Check sheet for the modelled part. Datum: model origin and axes. Units: mm. Face numbers are marked on the shaded views. A direction names the side the tool comes from. Coordinates: 2 decimals unless noted, no trailing zeros. Write each question's results on one line, items separated by ' | '. Start each with the question number.
1. Thickness scan on line 1 (Z direction, x = -0.5, y = -3.75); line 2 (X direction, y = 5, z = 14); line 3 (X direction, y = -1.5, z = 11). Record the ranges inside material, lowest first. Write a range as [from, to].
2. Gauge pin test, flat ends, axial feed: P1, Ø1, axis at y = -6, z = 10, coming from the +X side; P2, Ø1.5, axis at x = 7, y = 7.5, coming from the -Z side; P3, Ø1.5, axis at y = 6, z = 8.5, coming from the +X side. Record the tip position at first contact, or that the pin passes through.
3. Draft check along X on the marked faces 3, 4 and 5. Enter one of: released by +X, released by -X, zero draft, split by the parting line, or undercut.
4. Tool access check on the marked faces 1 and 2. Record the directions out of +Z, -Z, +X, -X, +Y, -Y that give a thin tool (end or side, any length) a straight path to the whole face; none if there is none.
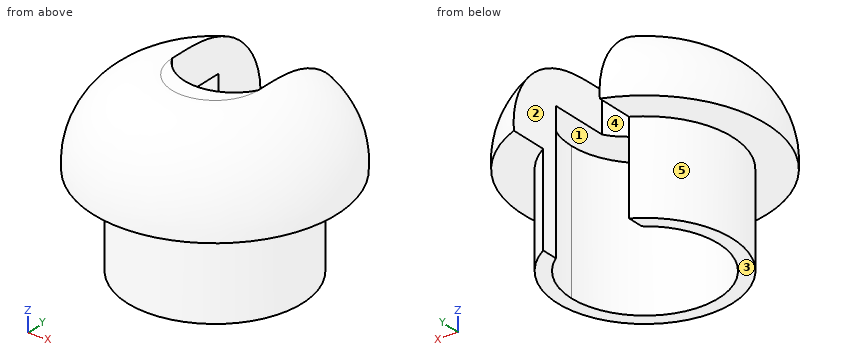
```python
from build123d import *

# Parameters (mm, degrees)
F4_DEPTH = 15.4777297208
F6_DEPTH = 12


with BuildPart() as f2:
    # F1 (on Front) → F2 (revolve)
    with BuildSketch(Plane.XZ):
        with BuildLine():
            Line((0, 15.4767297208), (0, 0))
            Line((0, 0), (7.625, 0))
            Line((7.625, 0), (7.625, 8))
            Line((7.625, 8), (10.625, 8))
            ThreePointArc((10.625, 8), (8.8302197506, 13.2471744611), (3.752507735, 15.4767297208))
            Line((3.752507735, 15.4767297208), (0, 15.4767297208))
        make_face()
    revolve(axis=Axis((0, 0, 0), (0, 0, 1)))

    # F3 (on face) → F4 (cut, through all)
    with BuildSketch(Plane.XY.offset(15.4767297208)):
        with BuildLine():
            ThreePointArc((-3.752507735, 0), (0, -2.1712493207), (3.752507735, 0))
            ThreePointArc((3.752507735, 0), (0, 3.752507735), (-3.752507735, 0))
        make_face()
        with BuildLine():
            Line((3.752507735, 0), (3.752507735, 9.9402872543))
            ThreePointArc((3.752507735, 9.9402872543), (0, 10.625), (-3.752507735, 9.9402872543))
            Line((-3.752507735, 9.9402872543), (-3.752507735, 0))
            ThreePointArc((-3.752507735, 0), (0, 3.752507735), (3.752507735, 0))
        make_face()
        with BuildLine():
            ThreePointArc((-3.752507735, 9.9402872543), (0, 10.625), (3.752507735, 9.9402872543))
            Line((3.752507735, 9.9402872543), (3.752507735, 12.1829835698))
            Line((3.752507735, 12.1829835698), (-3.752507735, 12.1829835698))
            Line((-3.752507735, 12.1829835698), (-3.752507735, 9.9402872543))
        make_face()
    extrude(amount=-F4_DEPTH, mode=Mode.SUBTRACT)

    # F5 (on face) → F6 (cut)
    with BuildSketch(Plane(origin=(0, 0, 0), x_dir=(1, 0, 0), z_dir=(0, 0, -1))):
        with BuildLine():
            ThreePointArc((3.752507735, -5.21529584), (5.7179754808, -2.9300821492), (6.425, 0))
            ThreePointArc((6.425, 0), (-2.9300821492, 5.7179754808), (-3.752507735, -5.21529584))
            Line((-3.752507735, -5.21529584), (-3.752507735, 0))
            ThreePointArc((-3.752507735, 0), (0, 2.1712493207), (3.752507735, 0))
            Line((3.752507735, 0), (3.752507735, -5.21529584))
        make_face()
        with BuildLine():
            Line((-3.752507735, 0), (-3.752507735, -5.21529584))
            ThreePointArc((-3.752507735, -5.21529584), (0, -6.425), (3.752507735, -5.21529584))
            Line((3.752507735, -5.21529584), (3.752507735, 0))
            ThreePointArc((3.752507735, 0), (0, 2.1712493207), (-3.752507735, 0))
        make_face()
    extrude(amount=-F6_DEPTH, mode=Mode.SUBTRACT)


solid = f2.part
```
Established:
1) line 1: [12, 15.48] | line 2: [-6.27, -3.75], [3.75, 6.27] | line 3: [-10.1, -6.25], [6.25, 10.1]
2) P1: x = 8.97 | P2: z = 8 | P3: x = 9.26
3) face 3: zero draft | face 4: undercut | face 5: split by the parting line
4) face 1: -Z | face 2: +Z, -Z, +Y
